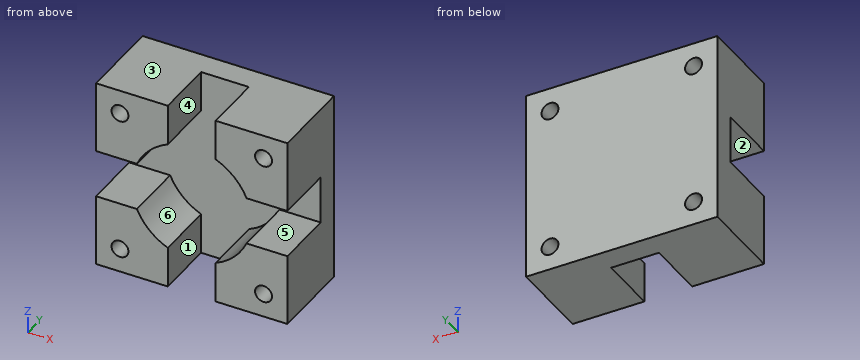
```python
from build123d import *

# Parameters (mm, degrees)
SKETCH1_W             = 50.8
SKETCH1_H             = 50.8
BOSS_EXTRUDE1_DEPTH   = 22.225
F_8_CLEARANCE_HOLE1_D = 4.4958
SKETCH9_W             = 12.7
SKETCH9_H             = 12.7
CUT_EXTRUDE1_DEPTH    = 15.875


with BuildPart() as part:
    # Sketch1 → Boss-Extrude1 (new body)
    with BuildSketch(Plane(origin=(0, 0, 0), x_dir=(1, 0, 0), z_dir=(0, 1, 0))):
        Rectangle(SKETCH1_W, SKETCH1_H)
    extrude(amount=BOSS_EXTRUDE1_DEPTH)

    # #8 Clearance Hole1 (through all)
    with Locations(Plane(origin=(0, 22.225, 0), x_dir=(1, 0, 0), z_dir=(0, 1, 0))):
        with Locations((-19.05, 19.05), (19.05, 19.05), (19.05, -19.05), (-19.05, -19.05)):
            Hole(F_8_CLEARANCE_HOLE1_D / 2)

    # Sketch9 → Cut-Extrude1 (cut)
    with BuildSketch(Plane.XZ):
        with BuildLine():
            ThreePointArc((-6.35, 14.549677831), (-11.225320151, 11.225320151), (-14.549677831, 6.35))
            Line((-14.549677831, 6.35), (-6.35, 6.35))
            Line((-6.35, 6.35), (-6.35, 14.549677831))
        make_face()
        with BuildLine():
            Line((-6.35, 25.4), (-6.35, 14.549677831))
            ThreePointArc((-6.35, 14.549677831), (0, 15.875), (6.35, 14.549677831))
            Line((6.35, 14.549677831), (6.35, 25.4))
            Line((6.35, 25.4), (-6.35, 25.4))
        make_face()
        with BuildLine():
            Line((6.35, 14.549677831), (6.35, 6.35))
            Line((6.35, 6.35), (14.549677831, 6.35))
            ThreePointArc((14.549677831, 6.35), (11.225320151, 11.225320151), (6.35, 14.549677831))
        make_face()
        with BuildLine():
            Line((25.4, 6.35), (14.549677831, 6.35))
            ThreePointArc((14.549677831, 6.35), (15.540137718, 3.243415594), (15.875, 0))
            ThreePointArc((15.875, 0), (15.540137718, -3.243415594), (14.549677831, -6.35))
            Line((14.549677831, -6.35), (25.4, -6.35))
            Line((25.4, -6.35), (25.4, 6.35))
        make_face()
        with BuildLine():
            Line((14.549677831, -6.35), (6.35, -6.35))
            Line((6.35, -6.35), (6.35, -14.549677831))
            ThreePointArc((6.35, -14.549677831), (11.225320151, -11.225320151), (14.549677831, -6.35))
        make_face()
        with BuildLine():
            ThreePointArc((6.35, -14.549677831), (0, -15.875), (-6.35, -14.549677831))
            Line((-6.35, -14.549677831), (-6.35, -25.4))
            Line((-6.35, -25.4), (6.35, -25.4))
            Line((6.35, -25.4), (6.35, -14.549677831))
        make_face()
        with BuildLine():
            Line((-6.35, -6.35), (-14.549677831, -6.35))
            ThreePointArc((-14.549677831, -6.35), (-11.225320151, -11.225320151), (-6.35, -14.549677831))
            Line((-6.35, -14.549677831), (-6.35, -6.35))
        make_face()
        with BuildLine():
            Line((-14.549677831, 6.35), (-25.4, 6.35))
            Line((-25.4, 6.35), (-25.4, -6.35))
            Line((-25.4, -6.35), (-14.549677831, -6.35))
            ThreePointArc((-14.549677831, -6.35), (-15.875, 0), (-14.549677831, 6.35))
        make_face()
        with BuildLine():
            Line((-6.35, 6.35), (-14.549677831, 6.35))
            ThreePointArc((-14.549677831, 6.35), (-15.875, 0), (-14.549677831, -6.35))
            Line((-14.549677831, -6.35), (-6.35, -6.35))
            Line((-6.35, -6.35), (-6.35, 6.35))
        make_face()
        with BuildLine():
            Line((6.35, -6.35), (-6.35, -6.35))
            Line((-6.35, -6.35), (-6.35, -14.549677831))
            ThreePointArc((-6.35, -14.549677831), (0, -15.875), (6.35, -14.549677831))
            Line((6.35, -14.549677831), (6.35, -6.35))
        make_face()
        with BuildLine():
            Line((14.549677831, 6.35), (6.35, 6.35))
            Line((6.35, 6.35), (6.35, -6.35))
            Line((6.35, -6.35), (14.549677831, -6.35))
            ThreePointArc((14.549677831, -6.35), (15.540137718, -3.243415594), (15.875, 0))
            ThreePointArc((15.875, 0), (15.540137718, 3.243415594), (14.549677831, 6.35))
        make_face()
        Rectangle(SKETCH9_W, SKETCH9_H)
        with BuildLine():
            Line((-6.35, 14.549677831), (-6.35, 6.35))
            Line((-6.35, 6.35), (6.35, 6.35))
            Line((6.35, 6.35), (6.35, 14.549677831))
            ThreePointArc((6.35, 14.549677831), (0, 15.875), (-6.35, 14.549677831))
        make_face()
    extrude(amount=-CUT_EXTRUDE1_DEPTH, mode=Mode.SUBTRACT)


solid = part.part
```
Work out the finished part from the listing and answer in its coordinate system (mm). Face numbers are marked on the shaded views. A direction names the side the tool comes from. Give positions to 0.01 mm unless a question says otherwise; leave off trailing zeros. Loops run counter-clockwise (first coordinate to the right, second up) from the corner with the lowest first, then second, coordinate; pieces in that order, holes last. Notation, with made-up numbers: (29, 83.25) - (45, 83.25) arc R34 cw to (45, 114.25) - close; hole circle Ø5 at (1, -9.75). An arc over 180 degrees is marked (long way). Use CSV: the item, a comma, the result in double quotes. Start each with the question number.
(1) A tool of negligible diameter and unlimited length cuts with its end or side. For the marked faces 4, 5 and 6, from which of +Z, -Z, +X, -X, +Y, -Y can it reach the whole face along a straight path? Write none if from no direction.
(2) Find section B-B, the plane z = -19.05. Determine the outline of the cut face in (x, y) (3 decimals), plus the area to 3 significant figures.
(3) Find the intervals of material crossed by L1, parallel to X at y = 6.75, z = -19.05; L2, parallel to Z at x = 19.05, y = 16, in increasing order.
(4) Find section D-D, the plane y = 19. Determine the outline of the cut face in (x, z).
(5) Find section A-A, the plane y = 10. Determine the outline of the cut face in (x, z) (3 decimals), plus the area to 3 significant figures.
(6) Determine the mould class of the marked faces 1, 2 and 3 for opening direction Z: released by +Z, released by -Z, zero draft, split by the parting line, or undercut.
(7) Find section C-C, the plane x = 18. Determine the outline of the cut face in (y, z) (3 decimals), plus the area to 3 significant figures.
(8) This flat-tipped pin is pushed along its axis until it touches: pin 1 (3.5 mm diameter, centred on x = -19.05, z = 19.05, fed in from -Y). Where does it stop, or does it pass through?
Results found:
1,face 4,"+Z, -Z, -Y"
1,face 5,"+X, -X, -Y"
1,face 6,"-Y"
2,outline,"(-25.4, 0) - (-21.298, 0) - (-21.298, 22.225) - (-25.4, 22.225) - close; (-16.802, 0) - (-6.35, 0) - (-6.35, 15.875) - (6.35, 15.875) - (6.35, 0) - (16.802, 0) - (16.802, 22.225) - (-16.802, 22.225) - close; (21.298, 0) - (25.4, 0) - (25.4, 22.225) - (21.298, 22.225) - close"
2,area,"728 mm^2"
3,L1,"-25.4 to -21.3, -16.8 to -6.35, 6.35 to 16.8, 21.3 to 25.4"
3,L2,"-25.4 to -21.3, -16.8 to 16.8, 21.3 to 25.4"
4,outline,"(-25.4, -25.4) - (25.4, -25.4) - (25.4, 25.4) - (-25.4, 25.4) - close; hole circle Ø4.5 at (-19.05, -19.05); hole circle Ø4.5 at (-19.05, 19.05); hole circle Ø4.5 at (19.05, -19.05); hole circle Ø4.5 at (19.05, 19.05)"
5,outline,"(-25.4, -25.4) - (-6.35, -25.4) - (-6.35, -14.55) arc R15.875 cw to (-14.55, -6.35) - (-25.4, -6.35) - close; (-25.4, 6.35) - (-14.55, 6.35) arc R15.875 cw to (-6.35, 14.55) - (-6.35, 25.4) - (-25.4, 25.4) - close; (6.35, -25.4) - (25.4, -25.4) - (25.4, -6.35) - (14.55, -6.35) arc R15.875 cw to (6.35, -14.55) - close; (6.35, 14.55) arc R15.875 cw to (14.55, 6.35) - (25.4, 6.35) - (25.4, 25.4) - (6.35, 25.4) - close; hole circle Ø4.496 at (-19.05, -19.05); hole circle Ø4.496 at (-19.05, 19.05); hole circle Ø4.496 at (19.05, -19.05); hole circle Ø4.496 at (19.05, 19.05)"
5,area,"1,220 mm^2"
6,face 1,"zero draft"
6,face 2,"undercut"
6,face 3,"released by +Z"
7,outline,"(0, -25.4) - (22.225, -25.4) - (22.225, -21.038) - (0, -21.038) - close; (0, -17.062) - (22.225, -17.062) - (22.225, 17.062) - (0, 17.062) - (0, 6.35) - (15.875, 6.35) - (15.875, -6.35) - (0, -6.35) - close; (0, 21.038) - (22.225, 21.038) - (22.225, 25.4) - (0, 25.4) - close"
7,area,"751 mm^2"
8,pin 1,"through"
